For this review, take the finished solid that the model builds, in its own axes (mm). Face numbers are marked on the shaded views. Coordinates: 2 decimals unless noted, no trailing zeros. Write each loop counter-clockwise with the first axis right and the second up, starting at its lowest first coordinate (ties: lowest second). Pieces come first, ordered by that corner, then holes. Notation, with made-up numbers: (-32, 59) -> (-4, 59) arc R15 cw to (-4, 88) -> close; hole circle Ø5 at (3.25, 84.5). An arc over 180 degrees is marked (long way). One line per item, written item: value. Start each with the question number.
1) Add section A-A (z = 10.5). State how many separate pieces and enclosed holes the cut face has, and give its area (3 significant figures).
2) Add section B-B (y = 8). State the section outline as (x, z) points (3 decimals).
3) Add section C-C (x = 33). State the section outline as (y, z) points (3 decimals).
4) For pin 1 Ø4.5 at (x, y) = (58, 34) entering from +Z (3 decimals); pin 2 Ø6.5 at (x, y) = (-58, -34) entering from -Z; pin 3 Ø5 at (x, z) = (-21.5, 10.5) entering from +Y; pin 4 Ø5 at (x, z) = (128.5, 4) entering from -Y, all flat-tipped, find the tip position at first contact; note any pin that passes through.
5) Mouldability with a two-part tool opening along X and no side actions: class the marked faces 1 and 2 as released by +X, released by -X, zero draft, split by the parting line, or undercut.
6) For probe 1 along X at (y, z) = (188.5, 12.5); probe 2 along Y at (x, z) = (22, 7.5); probe 3 along Y at (x, z) = (-58, 10), list the stretches that pass through material, from the lowest coordinate up. Write a range as from..to.
from build123d import *

# Parameters (mm, degrees)
SKETCH1_W           = 160
SKETCH1_H           = 144
SKETCH1_R           = 2.5
BOSS_EXTRUDE1_DEPTH = 15.875
BOSS_EXTRUDE2_DEPTH = 15.875
BOSS_EXTRUDE3_DEPTH = 15.875
FILLET2_R           = 10
SKETCH4_R           = 2.5
CUT_EXTRUDE1_DEPTH  = 314.466131544
FILLET3_R           = 1
SKETCH5_R           = 2.5
CUT_EXTRUDE2_DEPTH  = 314.466131544
FILLET4_R           = 2
SKETCH6_R           = 20
SKETCH6_R_2         = 2.5
CUT_EXTRUDE3_DEPTH  = 314.466131544
FILLET5_R           = 3


with BuildPart() as part:
    # Sketch1 → Boss-Extrude1 (new body)
    with BuildSketch(Plane.XY):
        Rectangle(SKETCH1_W, SKETCH1_H)
        with Locations((-58, -66)):
            Circle(SKETCH1_R, mode=Mode.SUBTRACT)
        with Locations((-22, -66)):
            Circle(SKETCH1_R, mode=Mode.SUBTRACT)
        with Locations((-58, -34)):
            Circle(SKETCH1_R, mode=Mode.SUBTRACT)
        with Locations((-22, -34)):
            Circle(SKETCH1_R, mode=Mode.SUBTRACT)
        with Locations(Location((58, -66, 0), (0, 0, 180))):
            Circle(SKETCH1_R, mode=Mode.SUBTRACT)
        with Locations(Location((22, -66, 0), (0, 0, 180))):
            Circle(SKETCH1_R, mode=Mode.SUBTRACT)
        with Locations(Location((22, -34, 0), (0, 0, 180))):
            Circle(SKETCH1_R, mode=Mode.SUBTRACT)
        with Locations(Location((58, -34, 0), (0, 0, 180))):
            Circle(SKETCH1_R, mode=Mode.SUBTRACT)
        with Locations(Location((-58, 66, 0), (0, 0, 180))):
            Circle(SKETCH1_R, mode=Mode.SUBTRACT)
        with Locations(Location((-22, 66, 0), (0, 0, 180))):
            Circle(SKETCH1_R, mode=Mode.SUBTRACT)
        with Locations((22, 66)):
            Circle(SKETCH1_R, mode=Mode.SUBTRACT)
        with Locations((58, 66)):
            Circle(SKETCH1_R, mode=Mode.SUBTRACT)
        with Locations((58, 34)):
            Circle(SKETCH1_R, mode=Mode.SUBTRACT)
        with Locations((22, 34)):
            Circle(SKETCH1_R, mode=Mode.SUBTRACT)
        with Locations(Location((-22, 34, 0), (0, 0, 180))):
            Circle(SKETCH1_R, mode=Mode.SUBTRACT)
        with Locations(Location((-58, 34, 0), (0, 0, 180))):
            Circle(SKETCH1_R, mode=Mode.SUBTRACT)
    extrude(amount=BOSS_EXTRUDE1_DEPTH)

    # Sketch2 → Boss-Extrude2 (add, through all)
    with BuildSketch(Plane.XY.offset(15.875)):
        Polygon((55, 272), (155, 272), (155, 152), (80, 152), (80, 72), (-80, 72), (-80, 122), align=None)
    extrude(amount=-BOSS_EXTRUDE2_DEPTH)

    # Sketch3 → Boss-Extrude3 (add, through all)
    with BuildSketch(Plane.XY.offset(15.875)):
        Polygon((155, 152), (80, 65.589776693), (80, 152), align=None)
    extrude(amount=-BOSS_EXTRUDE3_DEPTH)

    # Fillet2
    fillet2_edges = [part.edges().sort_by_distance(p)[0] for p in [
        (80, 65.589776693, 7.9375),
        (-80, 122, 7.9375),
        (55, 272, 7.9375),
    ]]
    fillet(fillet2_edges, radius=FILLET2_R)

    # Sketch4 → Cut-Extrude1 (cut, through all)
    with BuildSketch(Plane.XY.offset(15.875)):
        with Locations((-32, 20)):
            Circle(SKETCH4_R)
        with Locations(Location((-8, 20, 0), (0, 0, 180))):
            Circle(SKETCH4_R)
        with Locations((-8, -20)):
            Circle(SKETCH4_R)
        with Locations(Location((-32, -20, 0), (0, 0, 180))):
            Circle(SKETCH4_R)
    extrude(amount=-CUT_EXTRUDE1_DEPTH, mode=Mode.SUBTRACT)

    # Fillet3
    fillet3_edges = [part.edges().sort_by_distance(p)[0] for p in [
        (155, 272, 7.9375),
    ]]
    fillet(fillet3_edges, radius=FILLET3_R)

    # Sketch5 → Cut-Extrude2 (cut, through all)
    with BuildSketch(Plane.XY.offset(15.875)):
        with Locations((145, 262)):
            Circle(SKETCH5_R)
        with Locations((145, 242)):
            Circle(SKETCH5_R)
        with Locations((145, 222)):
            Circle(SKETCH5_R)
        with Locations((145, 202)):
            Circle(SKETCH5_R)
        with Locations((145, 182)):
            Circle(SKETCH5_R)
        with Locations((145, 162)):
            Circle(SKETCH5_R)
        with Locations((125, 162)):
            Circle(SKETCH5_R)
        with Locations((125, 262)):
            Circle(SKETCH5_R)
    extrude(amount=-CUT_EXTRUDE2_DEPTH, mode=Mode.SUBTRACT)

    # Fillet4
    fillet4_edges = [part.edges().sort_by_distance(p)[0] for p in [
        (155, 152, 7.9375),
    ]]
    fillet(fillet4_edges, radius=FILLET4_R)

    # Sketch6 → Cut-Extrude3 (cut, through all)
    with BuildSketch(Plane.XY.offset(15.875)):
        with Locations((105, 212)):
            Circle(SKETCH6_R)
        with Locations((81.5, 235.5)):
            Circle(SKETCH6_R_2)
        with Locations((128.5, 235.5)):
            Circle(SKETCH6_R_2)
        with Locations((128.5, 188.5)):
            Circle(SKETCH6_R_2)
        with Locations((81.5, 188.5)):
            Circle(SKETCH6_R_2)
    extrude(amount=-CUT_EXTRUDE3_DEPTH, mode=Mode.SUBTRACT)

    # Fillet5
    fillet5_edges = [part.edges().sort_by_distance(p)[0] for p in [
        (80, -72, 7.9375),
        (-80, -72, 7.9375),
    ]]
    fillet(fillet5_edges, radius=FILLET5_R)


solid = part.part
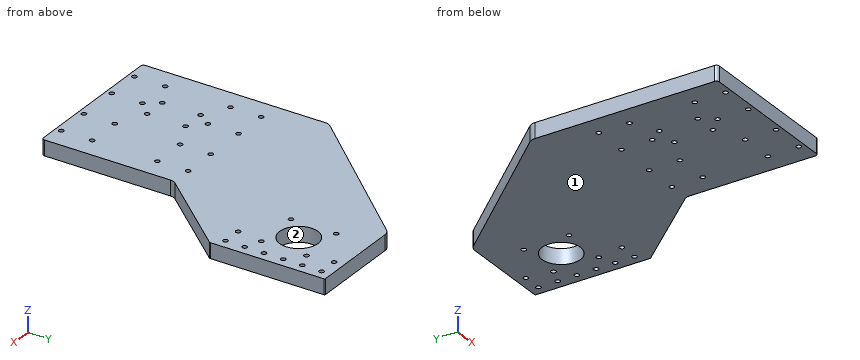
Numbers:
1. separate pieces: 1
1. enclosed holes: 33
1. area: 55,300 mm²
2. outline: (-80, 0) -> (80, 0) -> (80, 15.875) -> (-80, 15.875) -> close
3. outline: (-72, 0) -> (247.556, 0) -> (247.556, 15.875) -> (-72, 15.875) -> close
4. pin 1: through
4. pin 2: z = 0
4. pin 3: y = 189.78
4. pin 4: y = 118.59
5. face 1: zero draft
5. face 2: undercut
6. probe 1: -20.15..79, 84..126, 131..155
6. probe 2: -72..-68.5, -63.5..-36.5, -31.5..31.5, 36.5..63.5, 68.5..235.33
6. probe 3: -72..-68.5, -63.5..-36.5, -31.5..31.5, 36.5..63.5, 68.5..146.44
